from build123d import *

# Parameters (mm, degrees)
SKETCH_1_R          = 21
SKETCH_1_R_2        = 16
EXTRUDE_1_DEPTH     = 3
SKETCH_2_W          = 17.8
SKETCH_2_H          = 75
SKETCH_2_R          = 1.45
EXTRUDE_2_DEPTH     = 3
SKETCH_3_R          = 16
CUT_EXTRUDE_1_DEPTH = 91.034715527
FILLET_1_R          = 15


with BuildPart() as part:
    # 草图1 → 凸台-拉伸1 (new body)
    with BuildSketch(Plane.XY):
        Circle(SKETCH_1_R)
        Circle(SKETCH_1_R_2, mode=Mode.SUBTRACT)
    extrude(amount=EXTRUDE_1_DEPTH)

    # 草图2 → 凸台-拉伸2 (add)
    with BuildSketch(Plane.XY):
        with Locations((0, 50)):
            Rectangle(SKETCH_2_W, SKETCH_2_H)
        with Locations((0, 42.5)):
            Circle(SKETCH_2_R, mode=Mode.SUBTRACT)
        with Locations((0, 82.5)):
            Circle(SKETCH_2_R, mode=Mode.SUBTRACT)
    extrude(amount=EXTRUDE_2_DEPTH)

    # 草图3 → 切除-拉伸1 (cut, through all)
    with BuildSketch(Plane.XY.offset(3)):
        Circle(SKETCH_3_R)
    extrude(amount=-CUT_EXTRUDE_1_DEPTH, mode=Mode.SUBTRACT)

    # 圆角1
    fillet_1_edges = [part.edges().sort_by_distance(p)[0] for p in [
        (8.9, 19.020778112, 1.5),
        (-8.9, 19.020778112, 1.5),
    ]]
    fillet(fillet_1_edges, radius=FILLET_1_R)


solid = part.part
Could you check a few things on this model? Use its own coordinates, in mm. A direction names the side the tool comes from. Give positions to 0.01 mm unless a question says otherwise; leave off trailing zeros. Loops run counter-clockwise (first coordinate to the right, second up) from the corner with the lowest first, then second, coordinate; pieces in that order, holes last. Notation, with made-up numbers: (64, 82.25) -> (92, 82.25) arc R27 ccw to (92, 103.25) -> close; hole circle Ø11 at (-39, 48). An arc over 180 degrees is marked (long way). Return JSON: item names as keys, results as strings.
Item 1: If we section it at A-A on x = 0: List the corners of the cut face in (y, z) for me, plus the area to 3 significant figures.
Geometry results:
{"outline": "(-21, 0) -> (-16, 0) -> (-16, 3) -> (-21, 3) -> close; (16, 0) -> (41.05, 0) -> (41.05, 3) -> (16, 3) -> close; (43.95, 0) -> (81.05, 0) -> (81.05, 3) -> (43.95, 3) -> close; (83.95, 0) -> (87.5, 0) -> (87.5, 3) -> (83.95, 3) -> close", "area": "212 mm²"}
Item 2: If we section it at C-C on z = 0.9: List the corners of the cut face in (x, y) for me, plus the area to 3 significant figures.
Geometry results:
{"outline": "(-13.94, 15.7) arc R21 ccw (long way) to (13.94, 15.7) arc R15 cw to (8.9, 26.92) -> (8.9, 87.5) -> (-8.9, 87.5) -> (-8.9, 26.92) arc R15 cw to start; hole circle Ø32 at (0, 0); hole circle Ø2.9 at (0, 42.5); hole circle Ø2.9 at (0, 82.5)", "area": "1,780 mm²"}
Item 3: If we section it at D-D on y = 82.5: List the corners of the cut face in (x, z) for me, plus the area to 3 significant figures.
Geometry results:
{"outline": "(-8.9, 0) -> (-1.45, 0) -> (-1.45, 3) -> (-8.9, 3) -> close; (1.45, 0) -> (8.9, 0) -> (8.9, 3) -> (1.45, 3) -> close", "area": "44.7 mm²"}
Item 4: Which directions (+Z, -Z, +X, -X, +Y, -Y) give clear straight access to the entire face, cutting with the end or side of a thin tool? Please do faces 4 (the flat face through (-8.9, 57, 1)), 5 (the flat face through (0, 38, 0)).
Geometry results:
{"face 4": "+Z, -Z, -X, +Y", "face 5": "-Z, +X, -X, +Y, -Y"}
Item 5: We'd pull the mould along X, two halves only. Please class faces 1 (the cylindrical face through (-0.71, -20.988, 1.479)), 2 (the flat face through (8.9, 57, 1)), 3 (the cylindrical face through (13.314, 8.874, 1.479)): +X half, -X half, draft (parallel to the pull), parting line (faces both ways), or undercut.
Geometry results:
{"face 1": "parting line", "face 2": "+X half", "face 3": "undercut"}
Item 6: If we section it at B-B on y = 0: List the corners of the cut face in (x, z) for me, plus the area to 3 significant figures.
Geometry results:
{"outline": "(-21, 0) -> (-16, 0) -> (-16, 3) -> (-21, 3) -> close; (16, 0) -> (21, 0) -> (21, 3) -> (16, 3) -> close", "area": "30.0 mm²"}
Item 7: I need wall thicknesses on L1, parallel to Y at x = 0, z = 1.45; L2, parallel to X at y = 82.5, z = 1.05; L3, parallel to Y at x = -1, z = 2.05. Which ranges of each line are inside material? Lowest first, please. Write a range as from..to.
Geometry results:
{"L1": "y = -21..-16, 16..41.05, 43.95..81.05, 83.95..87.5", "L2": "x = -8.9..-1.45, 1.45..8.9", "L3": "y = -20.98..-15.97, 15.97..41.45, 43.55..81.45, 83.55..87.5"}
Item 8: I'm going to push flat-ended pins straight in: pin 1 (1 mm diameter, centred on x = -9, z = 2.5, fed in from -Y); pin 2 (1.5 mm diameter, centred on y = 46.5, z = 1.5, fed in from -X); pin 3 (12 mm diameter, centred on x = -3.5, y = 55.5, fed in from -Z). Where does each tip first touch, or does it pass through?
Geometry results:
{"pin 1": "stops at y = -19.2", "pin 2": "stops at x = -8.9", "pin 3": "stops at z = 0"}
